Part model, mm, in its own coordinate system. Face numbers are marked on the shaded views. Give positions to 0.01 mm unless a question says otherwise; leave off trailing zeros. Order: outer loops, then holes, each group sorted by start corner. A loop starts at its lowest first (then second) coordinate and runs counter-clockwise, first axis right, second up.
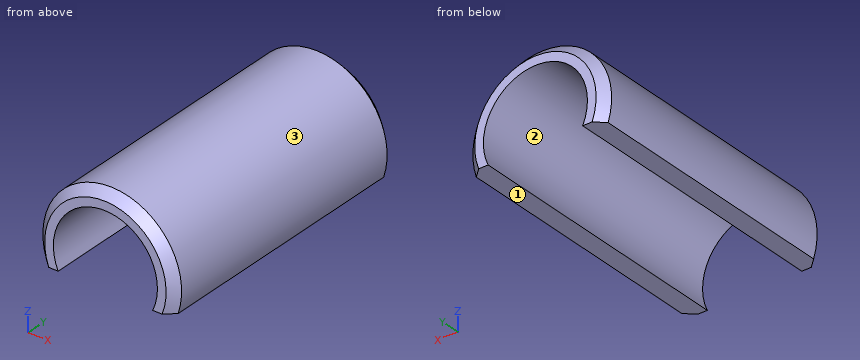
from build123d import *

# Parameters (mm, degrees)
BOX_W           = 100
BOX_H           = 100
BOX_DEPTH       = 100
TUBE001_R       = 16
TUBE001_R_2     = 12
TUBE001_DEPTH   = 64
CHAMFER003_SIZE = 2


with BuildPart() as krychle:
    # Box → Box (new body)
    with BuildSketch(Plane(origin=(32, -54, -63), x_dir=(1, 0, 0), z_dir=(0, 0, 1))):
        with Locations((50, 50)):
            Rectangle(BOX_W, BOX_H)
    extrude(amount=BOX_DEPTH)


with BuildPart() as cut381:
    # Tube001 → Tube001 (new body)
    with BuildSketch(Plane(origin=(75, 16, 42), x_dir=(1, 0, 0), z_dir=(0, -1, 0))):
        Circle(TUBE001_R)
        Circle(TUBE001_R_2, mode=Mode.SUBTRACT)
    extrude(amount=TUBE001_DEPTH)

    # Chamfer003
    chamfer003_edges = [cut381.edges().sort_by_distance(p)[0] for p in [
        (59, -48, 42),
        (59, 16, 42),
    ]]
    chamfer(chamfer003_edges, length=CHAMFER003_SIZE)

    # Cut381: cut Krychle
    add(krychle.part, mode=Mode.SUBTRACT)


solid = cut381.part
Item 1: Drill centre lines: probe 1 along X at (y, z) = (-30, 42); probe 2 along Z at (x, y) = (75, -6); probe 3 along X at (y, z) = (-29.5, 48.5). Where is each one in solid material? Low to high.
Item 2: Pull direction X, two halves, no side cores. Call the marked faces 1, 2 and 3: released by +X, released by -X, zero draft, split by the parting line, or undercut.
Item 3: Band-saw the part on B-B on x = 75. List the corners of the cut face in (y, z), plus the area to 3 significant figures.
Item 4: Band-saw the part on A-A on z = 42. List the corners of the cut face in (x, y).
Item 5: Drop flat-ended pins along their axis: P1, Ø6, axis at y = 2.5, z = 45, coming from the +X side; P2, Ø4, axis at x = 70, y = 8.5, coming from the -Z side; P3, Ø12, axis at x = 85.5, y = -41.5, coming from the +Z side; P4, Ø5, axis at x = 70, z = 48.5, coming from the -Y side. Give the stop position or say it passes through.
Item 6: Band-saw the part on C-C on y = -24.5. List the corners of the cut face in (x, z), plus the area to 3 significant figures.
Working result:
1. probe 1: x = 59 to 63, 87 to 91
1. probe 2: z = 54 to 58
1. probe 3: x = 60.38 to 64.91, 85.09 to 89.62
2. face 1: zero draft
2. face 2: undercut
2. face 3: split by the parting line
3. outline: (-48, 54) - (16, 54) - (16, 56) - (14, 58) - (-46, 58) - (-48, 56) - close
3. area: 252 mm2
4. outline: (59, -46) - (61, -48) - (63, -48) - (63, 16) - (61, 16) - (59, 14) - close; (87, -48) - (89, -48) - (91, -46) - (91, 14) - (89, 16) - (87, 16) - close
5. P1: stops at x = 91
5. P2: stops at z = 51.75
5. P3: stops at z = 57.35
5. P4: passes through
6. outline: (59.8, 37) - (64.09, 37) arc R12 cw (long way) to (85.91, 37) - (90.2, 37) arc R16 ccw (long way) to start
6. area: 217 mm2
